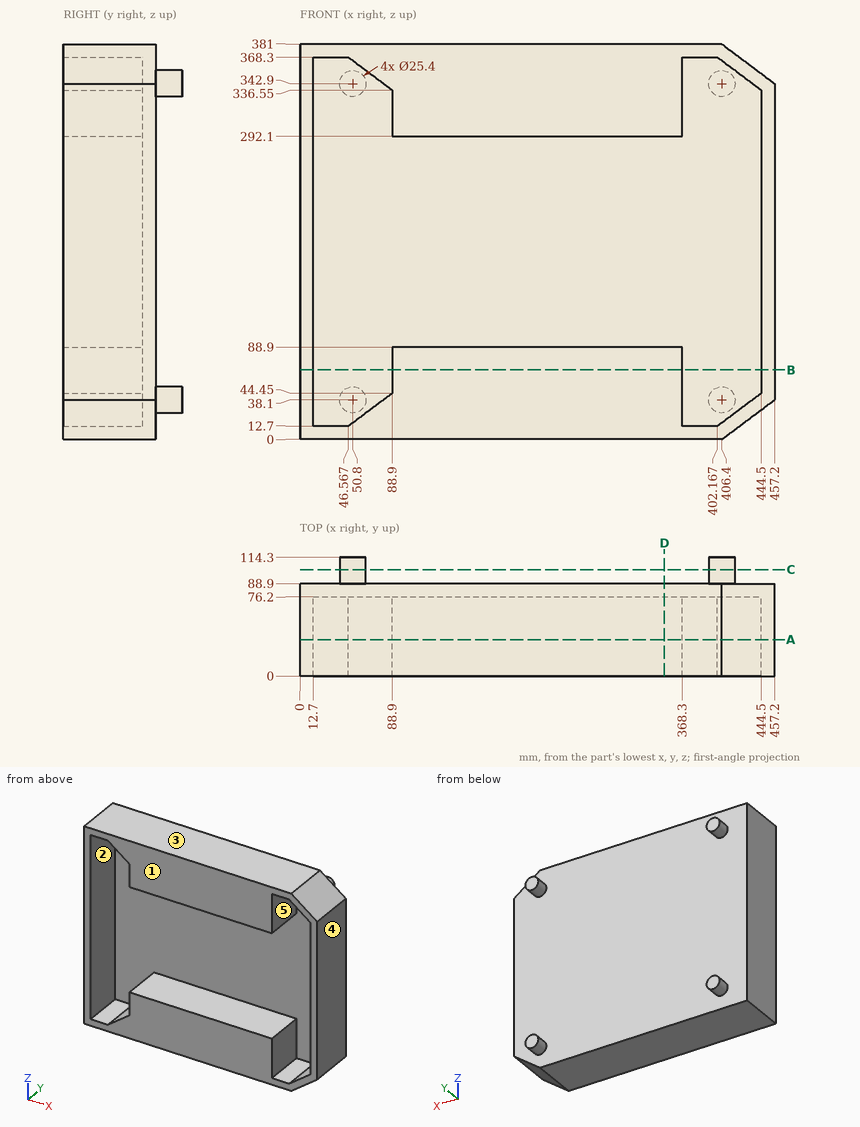
Answer from the drawing. Dimensions are ordinates in mm from the lowest x, y and z of the part. A direction names the side the tool comes from. Give positions to 0.01 mm unless a question says otherwise; leave off trailing zeros. Loops run counter-clockwise (first coordinate to the right, second up) from the corner with the lowest first, then second, coordinate; pieces in that order, holes last. Notation, with made-up numbers: (71.5, 52.25) - (87.5, 52.25) arc R11 cw to (87.5, 62.25) - close; hole circle Ø4 at (87.25, -2). An arc over 180 degrees is marked (long way). Answer as a JSON object with one key per item and string values.
1. Find the intervals of material crossed by L1, parallel to Z at x = 253.5, y = 68.5; L2, parallel to X at y = 27.5, z = 313.5; L3, parallel to X at y = 8, z = 271, in increasing order. Write a range as [from, to].
Determined:
{"L1": "[0, 88.9], [292.1, 381]", "L2": "[0, 12.7], [88.9, 368.3], [444.5, 457.2]", "L3": "[0, 12.7], [444.5, 457.2]"}
2. For the marked faces 1 and 2, determine the directions among +Z, -Z, +X, -X, +Y, -Y from which every point of the face is accessible in a straight line to the end or side of a thin tool.
Determined:
{"face 1": "+Z, -Z, +X, -X, -Y", "face 2": "-Y"}
3. A cutting plane is placed at A-A (y = 35). Write down the section's boundary in (x, z).
Determined:
{"outline": "(0, 0) - (406.4, 0) - (457.2, 38.1) - (457.2, 342.9) - (406.4, 381) - (0, 381) - close; hole (12.7, 12.7) - (46.57, 12.7) - (88.9, 44.45) - (88.9, 88.9) - (368.3, 88.9) - (368.3, 12.7) - (402.17, 12.7) - (444.5, 44.45) - (444.5, 336.55) - (402.17, 368.3) - (368.3, 368.3) - (368.3, 292.1) - (88.9, 292.1) - (88.9, 336.55) - (46.57, 368.3) - (12.7, 368.3) - close"}
4. Flat-ended cylindrical pins translate along their axes: pin 1 Ø1.5 at (x, z) = (339.5, 192.5) entering from +Y; pin 2 Ø4 at (x, z) = (293, 174.5) entering from -Y. Find the tip coordinate at first contact, or state that the pin passes through.
Determined:
{"pin 1": "y = 88.9", "pin 2": "y = 76.2"}
5. A cutting plane is placed at B-B (z = 67). Write down the section's boundary in (x, y).
Determined:
{"outline": "(0, 0) - (12.7, 0) - (12.7, 76.2) - (88.9, 76.2) - (88.9, 0) - (368.3, 0) - (368.3, 76.2) - (444.5, 76.2) - (444.5, 0) - (457.2, 0) - (457.2, 88.9) - (0, 88.9) - close"}
6. A cutting plane is placed at D-D (x = 351). Write down the section's boundary in (y, z), then the cut area to 3 significant figures.
Determined:
{"outline": "(0, 0) - (88.9, 0) - (88.9, 381) - (0, 381) - (0, 292.1) - (76.2, 292.1) - (76.2, 88.9) - (0, 88.9) - close", "area": "18,400 mm²"}
7. A cutting plane is placed at C-C (y = 102.5). Write down the section's boundary in (x, z), then the cut area to 3 significant figures.
Determined:
{"outline": "circle Ø25.4 at (50.8, 38.1); circle Ø25.4 at (50.8, 342.9); circle Ø25.4 at (406.4, 38.1); circle Ø25.4 at (406.4, 342.9)", "area": "2,030 mm²"}
8. For a pull along X with two mould halves and no side action, classify the marked faces 3, 4 and 5 as pulls with the +X half, pulls with the -X half, needs draft (parallel to the pull), parting line crosses it, or undercut.
Determined:
{"face 3": "needs draft", "face 4": "pulls with the +X half", "face 5": "undercut"}
